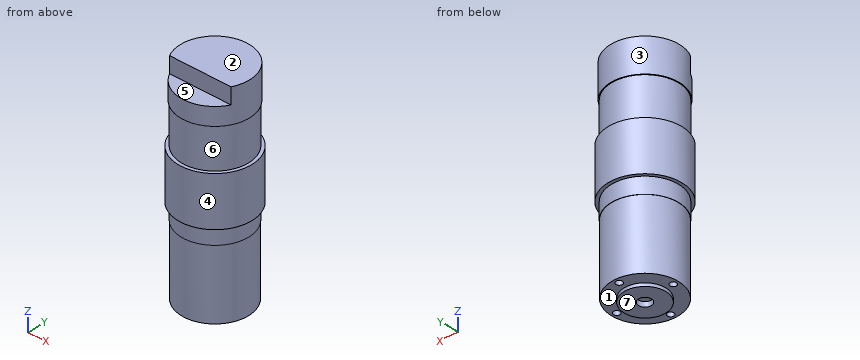
```python
from build123d import *

# Parameters (mm, degrees)
SKETCH1_R           = 21
BOSS_EXTRUDE1_DEPTH = 25
SKETCH2_R           = 23
BOSS_EXTRUDE2_DEPTH = 31
SKETCH3_R           = 21
BOSS_EXTRUDE3_DEPTH = 10
SKETCH4_R           = 20.85
BOSS_EXTRUDE4_DEPTH = 43.5
SKETCH5_R           = 13
BOSS_EXTRUDE5_DEPTH = 2
SKETCH6_R           = 4
CUT_EXTRUDE1_DEPTH  = 3
SKETCH7_R           = 21.5
BOSS_EXTRUDE6_DEPTH = 21
CUT_EXTRUDE2_START  = -10
CUT_EXTRUDE2_DEPTH  = 10
SKETCH9_R           = 2
CUT_EXTRUDE3_DEPTH  = 7


with BuildPart() as part:
    # Sketch1 → Boss-Extrude1 (new body)
    with BuildSketch(Plane.XY):
        Circle(SKETCH1_R)
    extrude(amount=-BOSS_EXTRUDE1_DEPTH)

    # Sketch2 → Boss-Extrude2 (add)
    with BuildSketch(Plane(origin=(0, 0, -25), x_dir=(-1, 0, 0), z_dir=(0, 0, -1))):
        Circle(SKETCH2_R)
    extrude(amount=BOSS_EXTRUDE2_DEPTH)

    # Sketch3 → Boss-Extrude3 (add)
    with BuildSketch(Plane(origin=(0, 0, -56), x_dir=(-1, 0, 0), z_dir=(0, 0, -1))):
        with Locations(Location((0, 0, 0), (0, 0, 180))):
            Circle(SKETCH3_R)
    extrude(amount=BOSS_EXTRUDE3_DEPTH)

    # Sketch4 → Boss-Extrude4 (add)
    with BuildSketch(Plane(origin=(0, 0, -66), x_dir=(-1, 0, 0), z_dir=(0, 0, -1))):
        Circle(SKETCH4_R)
    extrude(amount=BOSS_EXTRUDE4_DEPTH)

    # Sketch5 → Boss-Extrude5 (add)
    with BuildSketch(Plane(origin=(0, 0, -109.5), x_dir=(-1, 0, 0), z_dir=(0, 0, -1))):
        Circle(SKETCH5_R)
    extrude(amount=BOSS_EXTRUDE5_DEPTH)

    # Sketch6 → Cut-Extrude1 (cut)
    with BuildSketch(Plane(origin=(0, 0, -111.5), x_dir=(-1, 0, 0), z_dir=(0, 0, -1))):
        Circle(SKETCH6_R)
    extrude(amount=-CUT_EXTRUDE1_DEPTH, mode=Mode.SUBTRACT)

    # Sketch7 → Boss-Extrude6 (add)
    with BuildSketch(Plane.XY):
        with Locations(Location((0, 0, 0), (0, 0, 180))):
            Circle(SKETCH7_R)
    extrude(amount=BOSS_EXTRUDE6_DEPTH)

    # Sketch8 → Cut-Extrude2 (cut)
    with BuildSketch(Plane.XY.offset(21).offset(CUT_EXTRUDE2_START)):
        with BuildLine():
            Line((-19.032866311, -10), (19.032866311, -10))
            ThreePointArc((19.032866311, -10), (0, -21.5), (-19.032866311, -10))
        make_face()
    extrude(amount=CUT_EXTRUDE2_DEPTH, mode=Mode.SUBTRACT)

    # Sketch9 → Cut-Extrude3 (cut)
    with BuildSketch(Plane(origin=(0, 0, -109.5), x_dir=(-1, 0, 0), z_dir=(0, 0, -1))):
        with Locations((0, 17.5)):
            Circle(SKETCH9_R)
        with Locations((17.5, 0)):
            Circle(SKETCH9_R)
        with Locations((0, -17.5)):
            Circle(SKETCH9_R)
        with Locations((-17.5, 0)):
            Circle(SKETCH9_R)
    extrude(amount=-CUT_EXTRUDE3_DEPTH, mode=Mode.SUBTRACT)


solid = part.part
```
Can you work these out from the model? Positions are in its coordinate system, mm. Face numbers are marked on the shaded views. A direction names the side the tool comes from. Give positions to 0.01 mm unless a question says otherwise; leave off trailing zeros. Write each loop counter-clockwise with the first axis right and the second up, starting at its lowest first coordinate (ties: lowest second). Pieces come first, ordered by that corner, then holes. Notation, with made-up numbers: (6, -33.5) -> (64, -33.5) arc R15 cw to (64, -26.5) -> close; hole circle Ø2 at (-3.5, 13). An arc over 180 degrees is marked (long way). One line per item, written item: value.
Q1. We'd pull the mould along Z, two halves only. Please class the marked faces 4, 5, 6 and 7: +Z half, -Z half, draft (parallel to the pull), parting line (faces both ways), or undercut.
Results found:
face 4: draft
face 5: +Z half
face 6: undercut
face 7: -Z half
Q2. Which directions (+Z, -Z, +X, -X, +Y, -Y) give clear straight access to the entire face, cutting with the end or side of a thin tool? Please do the marked faces 1, 2 and 3.
Results found:
face 1: -Z
face 2: +Z, +X, -X, +Y, -Y
face 3: +Z
Q3. For P1, Ø2.5, axis at x = -1.5, y = 2, coming from the -Z side; P2, Ø12, axis at x = 5.5, z = -53.5, coming from the -Y side; P3, Ø2, axis at x = -1, y = 18, coming from the -Z side, each with a flat end and sliding along its axis, tell me the tip position at first contact or that it passes through.
Results found:
P1: stops at z = -108.5
P2: stops at y = -23
P3: stops at z = -109.5
Q4. Imagine slicing it at C-C on z = -59. Please give me the cut outline in (x, y), and give its area (3 significant figures).
Results found:
outline: circle Ø42 at (0, 0)
area: 1,390 mm^2
Q5. Imagine slicing it at A-A on y = 9. Please give me the cut outline in (x, z), and give its area (3 significant figures).
Results found:
outline: (-21.17, -56) -> (-18.97, -56) -> (-18.97, -66) -> (-18.81, -66) -> (-18.81, -109.5) -> (-9.38, -109.5) -> (-9.38, -111.5) -> (9.38, -111.5) -> (9.38, -109.5) -> (18.81, -109.5) -> (18.81, -66) -> (18.97, -66) -> (18.97, -56) -> (21.17, -56) -> (21.17, -25) -> (18.97, -25) -> (18.97, 0) -> (19.53, 0) -> (19.53, 21) -> (-19.53, 21) -> (-19.53, 0) -> (-18.97, 0) -> (-18.97, -25) -> (-21.17, -25) -> close
area: 5,130 mm^2
Q6. Imagine slicing it at D-D on y = -17.5. Please give me the cut outline in (x, z).
Results found:
outline: (-14.92, -56) -> (-11.61, -56) -> (-11.61, -66) -> (-11.33, -66) -> (-11.33, -109.5) -> (-2, -109.5) -> (-2, -102.5) -> (2, -102.5) -> (2, -109.5) -> (11.33, -109.5) -> (11.33, -66) -> (11.61, -66) -> (11.61, -56) -> (14.92, -56) -> (14.92, -25) -> (11.61, -25) -> (11.61, 0) -> (12.49, 0) -> (12.49, 11) -> (-12.49, 11) -> (-12.49, 0) -> (-11.61, 0) -> (-11.61, -25) -> (-14.92, -25) -> close
Q7. Imagine slicing it at B-B on x = -17.5. Please give me the cut outline in (y, z), and give its area (3 significant figures).
Results found:
outline: (-14.92, -56) -> (-11.61, -56) -> (-11.61, -66) -> (-11.33, -66) -> (-11.33, -109.5) -> (-2, -109.5) -> (-2, -102.5) -> (2, -102.5) -> (2, -109.5) -> (11.33, -109.5) -> (11.33, -66) -> (11.61, -66) -> (11.61, -56) -> (14.92, -56) -> (14.92, -25) -> (11.61, -25) -> (11.61, 0) -> (12.49, 0) -> (12.49, 21) -> (-10, 21) -> (-10, 11) -> (-12.49, 11) -> (-12.49, 0) -> (-11.61, 0) -> (-11.61, -25) -> (-14.92, -25) -> close
area: 3,200 mm^2
Q8. Please list where these lines run through material, in increasing order: line 1 (Y direction, x = 0, z = -104); line 2 (Y direction, x = 0, z = -109.25); line 3 (Z direction, x = -20.5, y = -5). Write a range as [from, to].
Results found:
line 1: y = [-20.85, -19.5], [-15.5, 15.5], [19.5, 20.85]
line 2: y = [-20.85, -19.5], [-15.5, -4], [4, 15.5], [19.5, 20.85]
line 3: z = [-56, -25], [0, 21]
